Geometry: final body of the model. Coordinates: model frame, mm. Give positions to 0.01 mm unless a question says otherwise; leave off trailing zeros. Loops run counter-clockwise (first coordinate to the right, second up) from the corner with the lowest first, then second, coordinate; pieces in that order, holes last. Notation, with made-up numbers: M 55.25,70 L 60.25,70 A21 cw 60.25,104 Z; hole C 46,76 d6. An arc over 180 degrees is marked long. Put each result on its own line as item: value.
```python
from build123d import *

# Parameters (mm, degrees)
EXTRUDE1_DEPTH             = 280
SKETCH2_R                  = 1.2
EXTRUDE2_DEPTH             = 4.8
SKETCH_R                   = 2.1
SKETCH_R_2                 = 1.2
EXTRUDE4_DEPTH             = 2.3
CHAMFER1_SIZE              = 0.2
LPATTERN1_COUNT            = 19
LPATTERN1_PITCH            = 15
CHAMFER1_OF_LPATTERN1_SIZE = 0.2


with BuildPart() as part:
    # Sketch1 → Extrude1 (new body)
    with BuildSketch(Plane.XY):
        with BuildLine():
            Line((-3.3, -2.4), (3.3, -2.4))
            Line((3.3, -2.4), (3.5, -2.2))
            Line((3.5, -2.2), (3.5, 0.106274607))
            ThreePointArc((3.5, 0.106274607), (3.091294745, 0.282570681), (2.840065792, 0.65))
            Line((2.840065792, 0.65), (2.340065792, 0.65))
            Line((2.340065792, 0.65), (2.340065792, 1.15))
            Line((2.340065792, 1.15), (2.840065792, 1.15))
            ThreePointArc((2.840065792, 1.15), (3.091294745, 1.517429319), (3.5, 1.693725393))
            Line((3.5, 1.693725393), (3.5, 2.2))
            Line((3.5, 2.2), (3.3, 2.4))
            Line((3.3, 2.4), (-3.3, 2.4))
            Line((-3.3, 2.4), (-3.5, 2.2))
            Line((-3.5, 2.2), (-3.5, 1.693725393))
            ThreePointArc((-3.5, 1.693725393), (-3.091294745, 1.517429319), (-2.840065792, 1.15))
            Line((-2.840065792, 1.15), (-2.340065792, 1.15))
            Line((-2.340065792, 1.15), (-2.340065792, 0.65))
            Line((-2.340065792, 0.65), (-2.840065792, 0.65))
            ThreePointArc((-2.840065792, 0.65), (-3.091294745, 0.282570681), (-3.5, 0.106274607))
            Line((-3.5, 0.106274607), (-3.5, -2.2))
            Line((-3.5, -2.2), (-3.3, -2.4))
        make_face()
    extrude(amount=EXTRUDE1_DEPTH)

    # Sketch2 → Extrude2 (cut)
    with BuildSketch(Plane(origin=(0, 2.4, 0), x_dir=(1, 0, 0), z_dir=(0, 1, 0))):
        with Locations((0, -5)):
            Circle(SKETCH2_R)
    extrude2 = extrude(amount=-EXTRUDE2_DEPTH, mode=Mode.SUBTRACT)

    # Sketch → Extrude4 (cut)
    with BuildSketch(Plane(origin=(0, 2.4, 0), x_dir=(1, 0, 0), z_dir=(0, 1, 0))):
        with Locations((0, -5)):
            Circle(SKETCH_R)
        with Locations((0, -5)):
            Circle(SKETCH_R_2, mode=Mode.SUBTRACT)
    extrude4 = extrude(amount=-EXTRUDE4_DEPTH, mode=Mode.SUBTRACT)

    # Chamfer1
    chamfer1_edges = [part.edges().sort_by_distance(p)[0] for p in [
        (-1.2, -2.4, 5),
        (-2.1, 2.4, 5),
    ]]
    chamfer(chamfer1_edges, length=CHAMFER1_SIZE)

    # LPattern1: Extrude2, Extrude4 ×19
    with Locations(*[(0, 0, i * LPATTERN1_PITCH) for i in range(1, LPATTERN1_COUNT)]):
        add(extrude2, mode=Mode.SUBTRACT)
        add(extrude4, mode=Mode.SUBTRACT)

    # Chamfer1 of LPattern1
    chamfer1_of_lpattern1_edges = [part.edges().sort_by_distance(p)[0] for p in [
        (-1.2, -2.4, 20),
        (-2.1, 2.4, 20),
        (-1.2, -2.4, 35),
        (-2.1, 2.4, 35),
        (-1.2, -2.4, 50),
        (-2.1, 2.4, 50),
        (-1.2, -2.4, 65),
        (-2.1, 2.4, 65),
        (-1.2, -2.4, 80),
        (-2.1, 2.4, 80),
        (-1.2, -2.4, 95),
        (-2.1, 2.4, 95),
        (-1.2, -2.4, 110),
        (-2.1, 2.4, 110),
        (-1.2, -2.4, 125),
        (-2.1, 2.4, 125),
        (-1.2, -2.4, 140),
        (-2.1, 2.4, 140),
        (-1.2, -2.4, 155),
        (-2.1, 2.4, 155),
        (-1.2, -2.4, 170),
        (-2.1, 2.4, 170),
        (-1.2, -2.4, 185),
        (-2.1, 2.4, 185),
        (-1.2, -2.4, 200),
        (-2.1, 2.4, 200),
        (-1.2, -2.4, 215),
        (-2.1, 2.4, 215),
        (-1.2, -2.4, 230),
        (-2.1, 2.4, 230),
        (-1.2, -2.4, 245),
        (-2.1, 2.4, 245),
        (-1.2, -2.4, 260),
        (-2.1, 2.4, 260),
        (-1.2, -2.4, 275),
        (-2.1, 2.4, 275),
    ]]
    chamfer(chamfer1_of_lpattern1_edges, length=CHAMFER1_OF_LPATTERN1_SIZE)


solid = part.part
```
Item 1: Pin query (flat end, axial travel): pin 1 Ø2.5 at (x, z) = (0, 20) entering from +Y. Return the tip coordinate at first contact, or that it passes through.
Output values:
pin 1: y = 0.1
Item 2: Line query: probe 1 along X at (y, z) = (-1.6, 65); probe 2 along X at (y, z) = (0.95, 185); probe 3 along Y at (x, z) = (2.5, 16). Output: solid intervals per line, ascending. Write a range as [from, to].
Output values:
probe 1: [-3.5, -1.2], [1.2, 3.5]
probe 2: [-2.34, -2.1], [2.1, 2.34]
probe 3: [-2.4, 0.65], [1.15, 2.4]
Item 3: Section B-B on y = -1.3. Count the separate pieces of the cut face and the enclosed holes in it, then the cut area to 3 significant figures.
Output values:
separate pieces: 1
enclosed holes: 19
area: 1,870 mm²
Item 4: Section A-A on z = 55. Output: boundary loops of the cut face in (x, y).
Output values:
outline: M -3.5,-2.2 L -3.3,-2.4 L 3.3,-2.4 L 3.5,-2.2 L 3.5,0.11 A0.8 cw 2.84,0.65 L 2.34,0.65 L 2.34,1.15 L 2.84,1.15 A0.8 cw 3.5,1.69 L 3.5,2.2 L 3.3,2.4 L -3.3,2.4 L -3.5,2.2 L -3.5,1.69 A0.8 cw -2.84,1.15 L -2.34,1.15 L -2.34,0.65 L -2.84,0.65 A0.8 cw -3.5,0.11 Z
